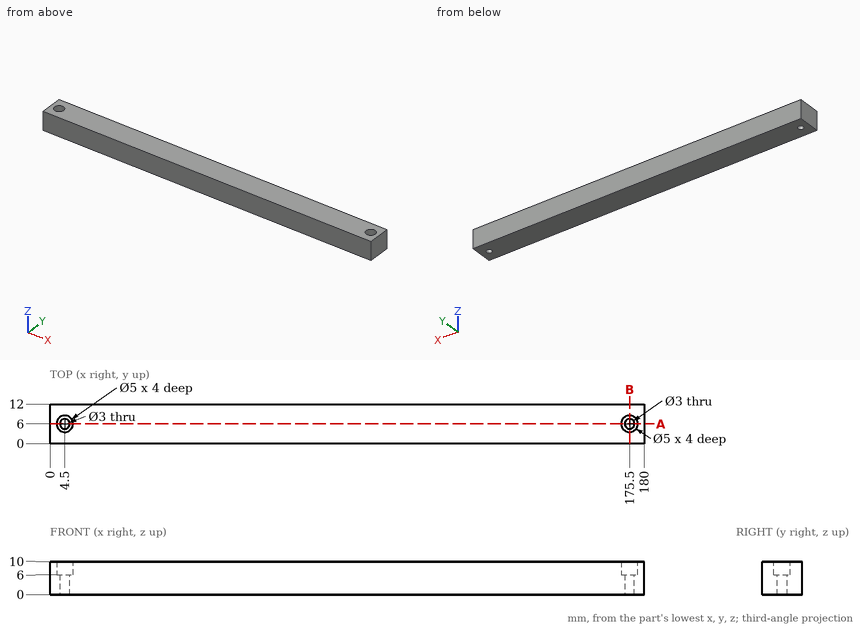
Drawing for the job (mm, zero at the part's lowest x, y, z). Round coordinates to 2 decimals unless told otherwise and drop trailing zeros. Loops run counter-clockwise (first coordinate to the right, second up) from the corner with the lowest first, then second, coordinate; pieces in that order, holes last. Notation, with made-up numbers: (3.5, 2.5) - (44.5, 2.5) arc R27 cw to (44.5, 32.5) - close; hole circle Ø3 at (74.5, -22). An arc over 180 degrees is marked (long way). Write each question's results on one line, items separated by ' | '.
(1) Wall check: L1, parallel to X at y = 6, z = 1.55; L2, parallel to X at y = 6, z = 8.05; L3, parallel to Y at x = 4.5, z = 2.05. Give the ranges that are in metal, low to high.
Answer below:
L1: x = 0 to 3, 6 to 174, 177 to 180 | L2: x = 0 to 2, 7 to 173, 178 to 180 | L3: y = 0 to 4.5, 7.5 to 12
(2) Pin check, flat tips, straight feed: pin 1 (3 mm diameter, centred on x = 160.5, z = 9, fed in from -Y); pin 2 (3.5 mm diameter, centred on x = 4.5, y = 6, fed in from +Z). Stop position of each tip, or through.
Answer below:
pin 1: stops at y = 0 | pin 2: stops at z = 6
(3) Saw through at A-A, the plane y = 6. List the corners of the cut face in (x, z), then the cut area to 3 significant figures.
Answer below:
outline: (0, 0) - (3, 0) - (3, 6) - (2, 6) - (2, 10) - (0, 10) - close; (6, 0) - (174, 0) - (174, 6) - (173, 6) - (173, 10) - (7, 10) - (7, 6) - (6, 6) - close; (177, 0) - (180, 0) - (180, 10) - (178, 10) - (178, 6) - (177, 6) - close | area: 1,720 mm^2
(4) Saw through at B-B, the plane x = 175.5. List the corners of the cut face in (y, z), then the cut area to 3 significant figures.
Answer below:
outline: (0, 0) - (4.5, 0) - (4.5, 6) - (3.5, 6) - (3.5, 10) - (0, 10) - close; (7.5, 0) - (12, 0) - (12, 10) - (8.5, 10) - (8.5, 6) - (7.5, 6) - close | area: 82.0 mm^2
